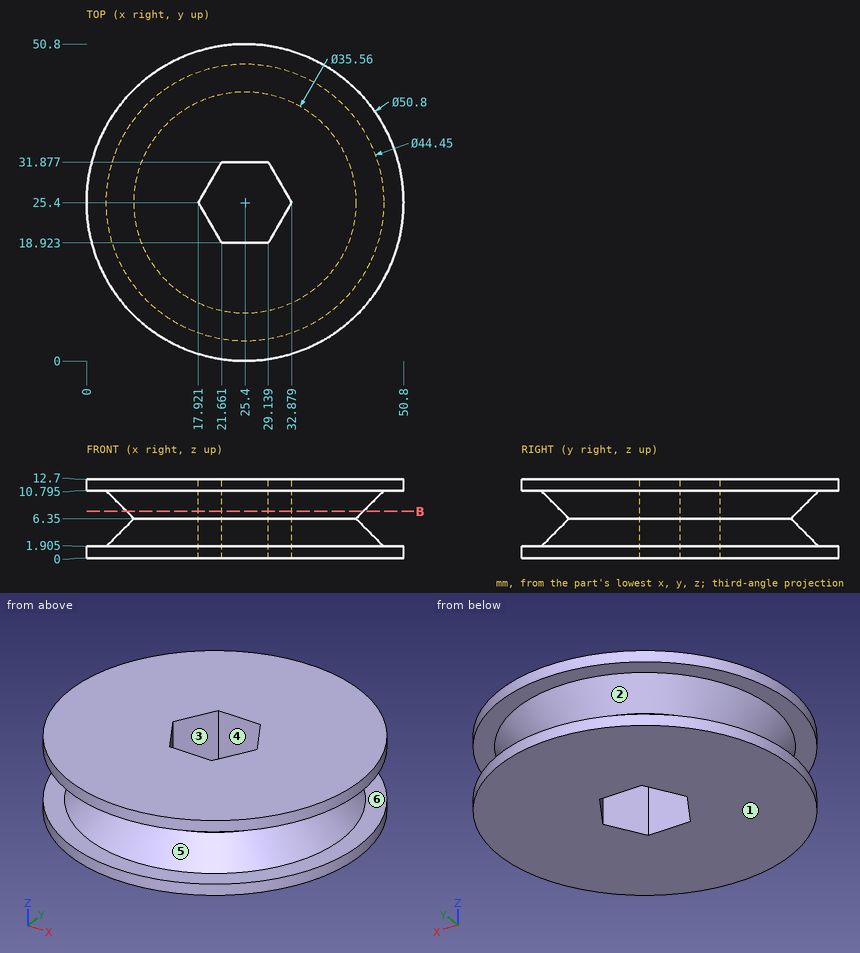
The drawing under review shows one solid part. Ordinate dimensions are in mm from its lowest x, y, z. A direction names the side the tool comes from. Round coordinates to 2 decimals unless told otherwise and drop trailing zeros. Write each loop counter-clockwise with the first axis right and the second up, starting at its lowest first coordinate (ties: lowest second). Pieces come first, ordered by that corner, then holes. Notation, with made-up numbers: (-21.5, 59.5) - (-17.5, 59.5) arc R21 ccw to (-17.5, 79.5) - close; hole circle Ø5 at (47, -8.75). An arc over 180 degrees is marked (long way). Put each result on its own line as item: value.
Q1. Insertion check: pin 1 Ø4 at (x, z) = (30, 4) entering from -Y (1 decimal); pin 2 Ø2 at (x, z) = (25, 8) entering from -Y (1 decimal); pin 3 Ø4 at (x, z) = (9.5, 5.5) entering from +Y. Each pin has a flat end and moves straight along its axis. Give the tip position at first contact, or say it passes through.
Solved:
pin 1: stops at y = 3.7
pin 2: stops at y = 5
pin 3: stops at y = 39.3
Q2. Wall thickness on probe 1 along Z at (x, y) = (17, 4) (1 decimal); probe 2 along X at (y, z) = (23, 11.5) (1 decimal); probe 3 along Z at (x, y) = (33, 42) (1 decimal): over which ranges is each line inside the solid? List them lowest first.
Solved:
probe 1: z = 0 to 1.9, 10.8 to 12.7
probe 2: x = 0.1 to 19.3, 31.5 to 50.7
probe 3: z = 0 to 5.9, 6.8 to 12.7
Q3. Machinability: for the marked faces 1, 2 and 3, which of the approach directions +Z, -Z, +X, -X, +Y, -Y give a long, thin tool a straight path to every point of the face, cutting with its end or side? Answer none if there is none.
Solved:
face 1: -Z, +X, -X, +Y, -Y
face 2: none
face 3: +Z, -Z
Q4. Mouldability with a two-part tool opening along X and no side actions: class the marked faces 4, 5 and 6 as released by +X, released by -X, zero draft, split by the parting line, or undercut.
Solved:
face 4: undercut
face 5: split by the parting line
face 6: zero draft
Q5. We need section B-B (z = 7.5). Give the boundary of the cut face in (x, y).
Solved:
outline: circle Ø37.86 at (25.4, 25.4); hole (17.92, 25.4) - (21.66, 18.92) - (29.14, 18.92) - (32.88, 25.4) - (29.14, 31.88) - (21.66, 31.88) - close
